Geometry: final body of the model. Coordinates: model frame, mm. A direction names the side the tool comes from. Give positions to 0.01 mm unless a question says otherwise; leave off trailing zeros. Loops run counter-clockwise (first coordinate to the right, second up) from the corner with the lowest first, then second, coordinate; pieces in that order, holes last. Notation, with made-up numbers: M 31,9.5 L 53,9.5 A21 ccw 53,25.5 Z; hole C 87,3 d5. An arc over 180 degrees is marked long. One line per question, with ' | ' between items. Start each with the question number.
from build123d import *

# Parameters (mm, degrees)
SKETCH5_W               = 20
SKETCH5_H               = 10
BOSS_EXTRUDE2_DEPTH     = 5
CUT_EXTRUDE2_DEPTH      = 13.247448714
CUT_EXTRUDE2_DEPTH_BACK = 13.247448714
SKETCH6_R               = 1.25
FILLET3_R               = 2
SKETCH7_W               = 1.25
SKETCH7_H               = 31


with BuildPart() as part:
    # Sketch5 → Boss-Extrude2 (new, symmetric)
    with BuildSketch(Plane.XY):
        Rectangle(SKETCH5_W, SKETCH5_H)
    extrude(amount=BOSS_EXTRUDE2_DEPTH, both=True)

    # Sketch6 → Cut-Extrude2 (cut, two sides: drawn at the far end of the back side and taken through both)
    with BuildSketch(Plane.XY.offset(-CUT_EXTRUDE2_DEPTH_BACK)):
        Circle(SKETCH6_R)
    extrude(amount=CUT_EXTRUDE2_DEPTH + CUT_EXTRUDE2_DEPTH_BACK, mode=Mode.SUBTRACT)

    # Fillet3
    fillet3_edges = [part.edges().sort_by_distance(p)[0] for p in [
        (10, 0, 5),
        (0, 5, 5),
        (-10, 0, 5),
        (0, 5, -5),
        (10, 0, -5),
        (0, -5, -5),
        (-10, 0, -5),
        (-10, 5, 0),
        (10, 5, 0),
        (10, -5, 0),
        (-10, -5, 0),
        (0, -5, 5),
    ]]
    fillet(fillet3_edges, radius=FILLET3_R)

    # Sketch7 → Revolve1 (revolve)
    with BuildSketch(Plane(origin=(0, 0, 0), x_dir=(1, 0, 0), z_dir=(0, 1, 0)), mode=Mode.PRIVATE) as revolve1_sk:
        with Locations((0.625, -10.5)):
            Rectangle(SKETCH7_W, SKETCH7_H)
    revolve(revolve1_sk.sketch.rotate(Axis((0, 0, -5), (0, 0, 1)), 180), axis=Axis((0, 0, -5), (0, 0, 1)))


solid = part.part
Q1. Section A-A, the plane x = 6.75. Output: boundary loops of the cut face in (y, z).
Q2. Material intervals for L1, parallel to Z at x = -4.5, y = -1.5; L2, parallel to Y at x = 0.5, z = 23.5, sorted ascending.
Q3. Contact query for flat-ended pins moving along their axis: pin 1 (6 mm diameter, centred on x = -4, z = 14, fed in from -Y); pin 2 (1 mm diameter, centred on y = -1.5, z = 9, fed in from +X); pin 3 (6 mm diameter, centred on y = -2, z = 18, fed in from +X). Output: stop coordinate, or through.
Q4. Section C-C, the plane y = 0. Output: boundary loops of the cut face in (x, z).
Q5. Section D-D, the plane x = 0. Output: boundary loops of the cut face in (y, z).
Q6. Section B-B, the plane z = 2. Output: boundary loops of the cut face in (x, y).
Q7. Set-up query: faces 1 (the cylindrical face through (-9.43, -4.4, 0.04)), 2 (the cylindrical face through (1.25, -0.05, 15.35)). Return all of +Z, -Z, +X, -X, +Y, -Y with unobstructed straight access to the full face (end or side cutting, diameter ignored); none if empty.
Model answer:
1) outline: M -5,-3 A2 ccw -3,-5 L 3,-5 A2 ccw 5,-3 L 5,3 A2 ccw 3,5 L -3,5 A2 ccw -5,3 Z
2) L1: z = -5 to 5 | L2: y = -1.15 to 1.15
3) pin 1: stops at y = -0.75 | pin 2: stops at x = 0.75 | pin 3: stops at x = 1.25
4) outline: M -10,-3 A2 ccw -8,-5 L 8,-5 A2 ccw 10,-3 L 10,3 A2 ccw 8,5 L 1.25,5 L 1.25,26 L -1.25,26 L -1.25,5 L -8,5 A2 ccw -10,3 Z
5) outline: M -5,-3 A2 ccw -3,-5 L 3,-5 A2 ccw 5,-3 L 5,3 A2 ccw 3,5 L 1.25,5 L 1.25,26 L -1.25,26 L -1.25,5 L -3,5 A2 ccw -5,3 Z
6) outline: M -10,-3 A2 ccw -8,-5 L 8,-5 A2 ccw 10,-3 L 10,3 A2 ccw 8,5 L -8,5 A2 ccw -10,3 Z
7) face 1: +Z, -Z, -X, -Y | face 2: +Z
